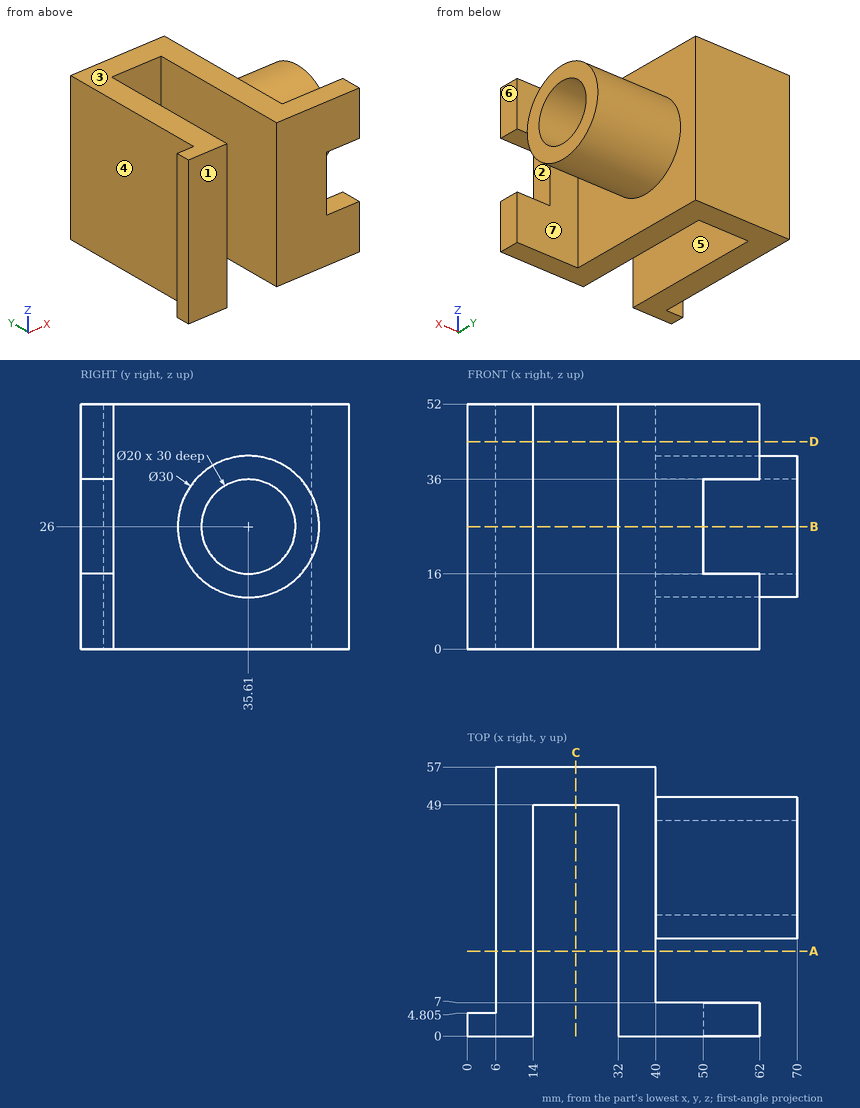
Answer from the drawing. Dimensions are ordinates in mm from the lowest x, y and z of the part. A direction names the side the tool comes from. Give positions to 0.01 mm unless a question says otherwise; leave off trailing zeros. Loops run counter-clockwise (first coordinate to the right, second up) from the corner with the lowest first, then second, coordinate; pieces in that order, holes last. Notation, with made-up numbers: (27.25, 85) - (71.25, 85) arc R12 ccw to (71.25, 90) - close; hole circle Ø4 at (13.25, 57). An arc over 180 degrees is marked (long way). Write each question's results on one line, items separated by ' | '.
1. Find section D-D, the plane z = 44. Write down the section's boundary in (x, y) (1 decimal), then the cut area to 3 significant figures.
Resolved:
outline: (0, 0) - (14, 0) - (14, 49) - (32, 49) - (32, 0) - (62, 0) - (62, 7) - (40, 7) - (40, 57) - (6, 57) - (6, 4.8) - (0, 4.8) - close | area: 1,240 mm^2
2. Flat-ended cylindrical pins translate along their axes: P1, Ø4, axis at x = 28.5, y = 24, coming from the -Z side; P2, Ø5, axis at y = 46.5, z = 14.5, coming from the -X side; P3, Ø5.5, axis at x = 23, z = 25.5, coming from the -Y side; P4, Ø3, axis at x = 4, z = 35.5, coming from the +Y side (1 decimal). Find the tip coordinate at first contact, or state that the pin passes through.
Resolved:
P1: passes through | P2: stops at x = 6 | P3: stops at y = 49 | P4: stops at y = 4.8
3. For a pull along Z with two mould halves and no side action, classify the marked faces 1, 2 and 3 as +Z half, -Z half, draft (parallel to the pull), parting line (faces both ways), or undercut.
Resolved:
face 1: draft | face 2: undercut | face 3: +Z half
4. Find section B-B, the plane z = 26. Write down the section's boundary in (x, y) (1 decimal).
Resolved:
outline: (0, 0) - (14, 0) - (14, 49) - (32, 49) - (32, 0) - (50, 0) - (50, 7) - (40, 7) - (40, 20.6) - (70, 20.6) - (70, 25.6) - (40, 25.6) - (40, 45.6) - (70, 45.6) - (70, 50.6) - (40, 50.6) - (40, 57) - (6, 57) - (6, 4.8) - (0, 4.8) - close
5. Find section A-A, the plane y = 18. Write down the section's boundary in (x, z).
Resolved:
outline: (6, 0) - (14, 0) - (14, 52) - (6, 52) - close; (32, 0) - (40, 0) - (40, 52) - (32, 52) - close
6. Find section C-C, the plane x = 23. Write down the section's boundary in (y, z), then the cut area to 3 significant figures.
Resolved:
outline: (49, 0) - (57, 0) - (57, 52) - (49, 52) - close | area: 416 mm^2
7. Which of the six approach directions +Z, -Z, +X, -X, +Y, -Y give full straight-line access (tool end or side, diameter ignored) to the marked faces 4, 5, 6 and 7?
Resolved:
face 4: +Z, -Z, -X, +Y | face 5: +Z, -Z, -Y | face 6: +Z, -Z, +X, -Y | face 7: +Z, -Z, +X
8. Consider probe 1 along Y at (x, z) = (48, 26); probe 2 along Y at (x, z) = (63.5, 26); probe 3 along X at (y, z) = (21.5, 12). Determine where each line is inside the solid, lowest interval first. Write a range as from..to.
Resolved:
probe 1: y = 0..7, 20.61..25.61, 45.61..50.61 | probe 2: y = 20.61..25.61, 45.61..50.61 | probe 3: x = 6..14, 32..40
